Design review of the part built by this model. Coordinates are the model's own, in mm. A direction names the side the tool comes from. Give positions to 0.01 mm unless a question says otherwise; leave off trailing zeros. Order: outer loops, then holes, each group sorted by start corner. A loop starts at its lowest first (then second) coordinate and runs counter-clockwise, first axis right, second up. Notation, with made-up numbers: (6.5, 29) - (44.5, 29) arc R11 cw to (44.5, 38) - close; hole circle Ø9 at (68, 21.5). An arc over 180 degrees is marked (long way). Write each question's results on one line, items separated by ' | '. Start each with the question number.
```python
from build123d import *

# Parameters (mm, degrees)
CYLINDER013_R     = 13.9827
CYLINDER013_DEPTH = 64.36
CYLINDER011_R     = 13.9827
CYLINDER011_DEPTH = 64.36
CYLINDER012_R     = 13.9827
CYLINDER012_DEPTH = 31.877


with BuildPart() as cylinder013:
    # Cylinder013 → Cylinder013 (new body)
    with BuildSketch(Plane(origin=(0, 0, -32.18), x_dir=(0, 1, 0), z_dir=(0, 0, 1))):
        Circle(CYLINDER013_R)
    extrude(amount=CYLINDER013_DEPTH)


with BuildPart() as cylinder011:
    # Cylinder011 → Cylinder011 (new body)
    with BuildSketch(Plane.XZ.offset(-32.1818)):
        Circle(CYLINDER011_R)
    extrude(amount=CYLINDER011_DEPTH)


with BuildPart() as f_5_way:
    # Cylinder012 → Cylinder012 (new body)
    with BuildSketch(Plane(origin=(0, 0, 0), x_dir=(0, 0, -1), z_dir=(1, 0, 0))):
        Circle(CYLINDER012_R)
    extrude(amount=CYLINDER012_DEPTH)

    # Fusion005: union Cylinder013, Cylinder011
    add(cylinder013.part)
    add(cylinder011.part)


solid = f_5_way.part
```
Q1. For line 1 (Z direction, x = 0, y = -23.5); line 2 (Y direction, x = 14.5, z = 0.5), list the stretches that pass through material, from the lowest coordinate up. Write a range as [from, to].
Q2. Draft analysis for pull direction Y (two halves, no side actions). For faces 6 (the flat face through (0, -32.178, 0)), 7 (the flat face through (0, 32.182, 0)), 8 (the cylindrical face through (-13.864, -1.82, -19.891)), 9 (the flat face through (31.877, 0, 0)), state which applies: pulls with the +Y half, pulls with the -Y half, needs draft (parallel to the pull), parting line crosses it, or undercut.
Q3. Insertion check: pin 1 Ø5 at (x, z) = (3.5, 20.5) entering from -Y; pin 2 Ø4 at (x, y) = (6.5, -20.5) entering from -Z; pin 3 Ø10 at (y, z) = (9.5, 24.5) entering from -X. Each pin has a flat end and moves straight along its axis. Give the tip position at first contact, or say it passes through.
Q4. Machinability: for faces 1 (the cylindrical face through (-13.97, -19.44, 0.61)), 2 (the cylindrical face through (23.2, 11.8, -7.5)), 3 (the flat face through (0, 0, 32.18)), 4 (the cylindrical face through (-13.97, 19.89, 0.61)), 5 (the cylindrical face through (-13.864, -1.82, 23.016)), which of the approach directions +Z, -Z, +X, -X, +Y, -Y give a long, thin tool a straight path to every point of the face, cutting with its end or side? Answer none if there is none.
Q5. Add section C-C (y = 16). Give the boundary of the cut face in (x, z).
Q6. Add section A-A (x = 0). Give the boundary of the cut face in (y, z), plus the area to 3 significant figures.
Q7. Add section B-B (z = -12). Give the boundary of the cut face in (x, y).
Verdict:
1) line 1: z = [-13.98, 13.98] | line 2: y = [-13.97, 13.97]
2) face 6: pulls with the -Y half | face 7: pulls with the +Y half | face 8: parting line crosses it | face 9: needs draft
3) pin 1: stops at y = -13.95 | pin 2: stops at z = -13.24 | pin 3: stops at x = -13.24
4) face 1: -Y | face 2: +X | face 3: +Z, +X, -X, +Y, -Y | face 4: +Y | face 5: +Z
5) outline: circle Ø27.97 at (0, 0)
6) outline: (-32.18, -13.98) - (-13.98, -13.98) - (-13.98, -32.18) - (13.98, -32.18) - (13.98, -13.98) - (32.18, -13.98) - (32.18, 13.98) - (13.98, 13.98) - (13.98, 32.18) - (-13.98, 32.18) - (-13.98, 13.98) - (-32.18, 13.98) - close | area: 2,820 mm2
7) outline: (-7.18, -32.18) - (7.18, -32.18) - (7.18, -12) arc R13.98 ccw to (12, -7.18) - (31.88, -7.18) - (31.88, 7.18) - (12, 7.18) arc R13.98 ccw to (7.18, 12) - (7.18, 32.18) - (-7.18, 32.18) - (-7.18, 12) arc R13.98 ccw to (-7.18, -12) - close
